Source: CAD feature listing. Evaluate the final solid. Frame: model axes, mm. Face numbers are marked on the shaded views. A direction names the side the tool comes from. Coordinates: 2 decimals unless noted, no trailing zeros. Write each loop counter-clockwise with the first axis right and the second up, starting at its lowest first coordinate (ties: lowest second). Pieces come first, ordered by that corner, then holes. Notation, with made-up numbers: (59, 83) -> (98, 83) arc R12 cw to (98, 104) -> close; hole circle Ø4 at (37, -23). An arc over 180 degrees is marked (long way). One line per item, written item: value. Start each with the question number.
1. Section query A-A, the plane x = -35. Output: boundary loops of the cut face in (y, z), and give its area (3 significant figures).
2. First-contact query: P1, Ø12, axis at x = -37, z = 20.5, coming from the +Y side; P2, Ø16, axis at x = -35, z = 35, coming from the -Y side. Flat tips, straight axial feed; report the tip coordinate or a pass-through.
3. Access query for the marked faces 1 and 2. Directions: +Z, -Z, +X, -X, +Y, -Y. A direction counts if a zero-diameter tool reaches every point of the face in a straight line with its end or side. Return the directions, or none.
4. Mould query, pull axis X, two halves, no side actions, for the marked faces 3, 4 and 5. Classes: released by +X, released by -X, zero draft, split by the parting line, or undercut.
5. Line query: line 1 (Z direction, x = -35, y = -8); line 2 (Z direction, x = -11, y = -12); line 3 (X direction, y = -13, z = 0). Output: solid intervals per line, ascending.
6. Section query C-C, the plane y = -8.5. Output: boundary loops of the cut face in (x, z).
7. Section query B-B, the plane z = 35. Output: boundary loops of the cut face in (x, y), and give its area (3 significant figures).
from build123d import *

# Parameters (mm, degrees)
F0_W     = 100
F0_H     = 100
F1_DEPTH = 15
F2_R     = 10
F3_DEPTH = 15.001
F4_SIZE  = 5


with BuildPart() as f1:
    # F0 (on Front) → F1 (new body)
    with BuildSketch(Plane.XZ):
        Rectangle(F0_W, F0_H)
        Polygon((15, 25.980762), (30, 0), (15, -25.980762), (-15, -25.980762), (-30, 0), (-15, 25.980762), align=None, mode=Mode.SUBTRACT)
    extrude(amount=F1_DEPTH)

    # F2 (on face) → F3 (cut, through all)
    with BuildSketch(Plane.XZ.offset(15)):
        with Locations((-35, 35)):
            Circle(F2_R)
    extrude(amount=-F3_DEPTH, mode=Mode.SUBTRACT)

    # F4
    f4_edges = [f1.edges().sort_by_distance(p)[0] for p in [
        (50, -7.5, 50),
        (-50, -7.5, 50),
        (50, -7.5, -50),
        (-50, -7.5, -50),
    ]]
    chamfer(f4_edges, length=F4_SIZE)


solid = f1.part
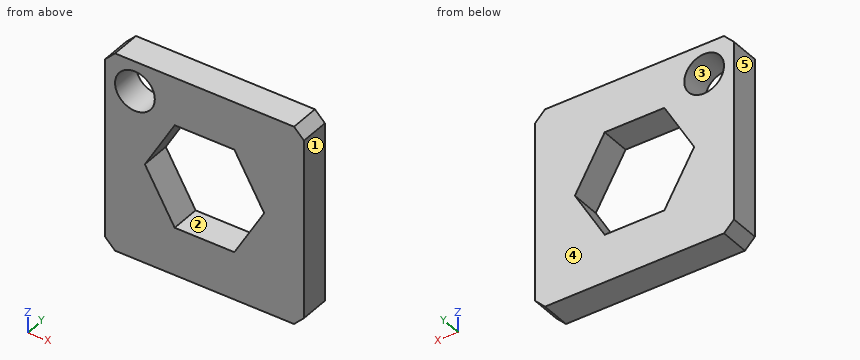
Computed values:
1. outline: (-15, -50) -> (0, -50) -> (0, 25) -> (-15, 25) -> close; (-15, 45) -> (0, 45) -> (0, 50) -> (-15, 50) -> close
1. area: 1,200 mm²
2. P1: stops at y = 0
2. P2: passes through
3. face 1: +Z, -Z, +X, +Y, -Y
3. face 2: +Y, -Y
4. face 3: undercut
4. face 4: zero draft
4. face 5: released by -X
5. line 1: z = -50 to 25, 45 to 50
5. line 2: z = -50 to -25.98, 25.98 to 50
5. line 3: x = -50 to -30, 30 to 50
6. outline: (-50, -45) -> (-45, -50) -> (45, -50) -> (50, -45) -> (50, 45) -> (45, 50) -> (-45, 50) -> (-50, 45) -> close; hole circle Ø20 at (-35, 35); hole (-30, 0) -> (-15, -25.98) -> (15, -25.98) -> (30, 0) -> (15, 25.98) -> (-15, 25.98) -> close
7. outline: (-50, -15) -> (-45, -15) -> (-45, 0) -> (-50, 0) -> close; (-25, -15) -> (50, -15) -> (50, 0) -> (-25, 0) -> close
7. area: 1,200 mm²
